For this review, take the finished solid that the model builds, in its own axes (mm). Face numbers are marked on the shaded views. A direction names the side the tool comes from. Round coordinates to 2 decimals unless told otherwise and drop trailing zeros. Write each loop counter-clockwise with the first axis right and the second up, starting at its lowest first coordinate (ties: lowest second). Pieces come first, ordered by that corner, then holes.
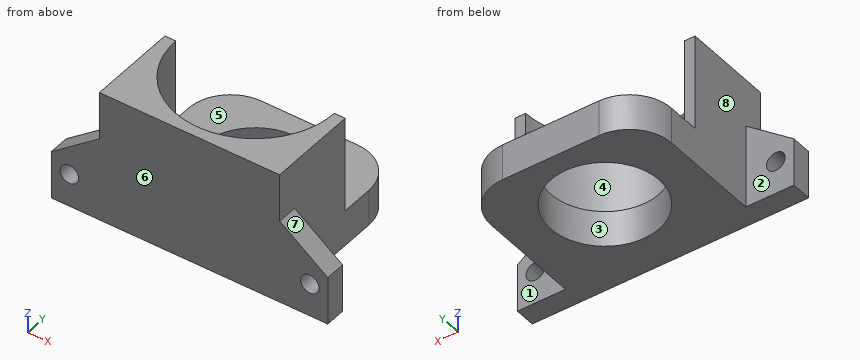
from build123d import *

# Parameters (mm, degrees)
BOSS_EXTRUDE1_DEPTH = 6
SKETCH2_R           = 9
CUT_EXTRUDE1_DEPTH  = 6
FILLET1_R           = 7
BOSS_EXTRUDE2_DEPTH = 16
SKETCH5_W           = 8
SKETCH5_H           = 3.4
BOSS_EXTRUDE3_DEPTH = 2
SKETCH6_R           = 1.55
CUT_EXTRUDE3_DEPTH  = 40.862262856
BOSS_EXTRUDE5_DEPTH = 3.4


with BuildPart() as part:
    # Sketch1 → Boss-Extrude1 (new body)
    with BuildSketch(Plane.XY):
        Polygon((-23, 0), (23, 0), (23, 3.4), (15, 3.4), (15, 27.4), (-15, 27.4), (-15, 3.4), (-23, 3.4), align=None)
    extrude(amount=BOSS_EXTRUDE1_DEPTH)

    # Sketch2 → Cut-Extrude1 (cut)
    with BuildSketch(Plane(origin=(0, 0, 0), x_dir=(-1, 0, 0), z_dir=(0, 0, -1))):
        with Locations((0, 15)):
            Circle(SKETCH2_R)
    extrude(amount=-CUT_EXTRUDE1_DEPTH, mode=Mode.SUBTRACT)

    # Fillet1
    fillet1_edges = [part.edges().sort_by_distance(p)[0] for p in [
        (-15, 27.4, 3),
        (15, 27.4, 3),
    ]]
    fillet(fillet1_edges, radius=FILLET1_R)

    # Sketch4 → Boss-Extrude2 (add)
    with BuildSketch(Plane.XY.offset(6)):
        with BuildLine():
            Line((-15, 0), (15, 0))
            Line((15, 0), (15, 15))
            Line((15, 15), (13.2, 15))
            ThreePointArc((13.2, 15), (0, 1.8), (-13.2, 15))
            Line((-13.2, 15), (-15, 15))
            Line((-15, 15), (-15, 0))
        make_face()
    extrude(amount=BOSS_EXTRUDE2_DEPTH)

    # Sketch5 → Boss-Extrude3 (add)
    with BuildSketch(Plane.XY.offset(6)):
        with Locations((-19, 1.7)):
            Rectangle(SKETCH5_W, SKETCH5_H)
        with Locations((19, 1.7)):
            Rectangle(SKETCH5_W, SKETCH5_H)
    extrude(amount=BOSS_EXTRUDE3_DEPTH)

    # Sketch6 → Cut-Extrude3 (cut, through all)
    with BuildSketch(Plane(origin=(0, 3.4, 0), x_dir=(1, 0, 0), z_dir=(0, 1, 0))):
        with Locations(Location((20, -5.5, 0), (0, 0, 270))):
            Circle(SKETCH6_R)
        with Locations(Location((-20, -5.5, 0), (0, 0, 270))):
            Circle(SKETCH6_R)
    extrude(amount=-CUT_EXTRUDE3_DEPTH, mode=Mode.SUBTRACT)

    # Sketch8 → Boss-Extrude5 (add)
    with BuildSketch(Plane(origin=(0, 0, 0), x_dir=(1, 0, 0), z_dir=(0, 1, 0))):
        Polygon((-23, -8), (-15, -14), (-15, -8), align=None)
        Polygon((15, -14), (23, -8), (15, -8), align=None)
    extrude(amount=BOSS_EXTRUDE5_DEPTH)


solid = part.part
(1) We need section D-D, the plane z = 11. Give the boundary of the cut face in (x, y).
Geometry check:
outline: (-19, 0) - (19, 0) - (19, 3.4) - (15, 3.4) - (15, 15) - (13.2, 15) arc R13.2 cw to (-13.2, 15) - (-15, 15) - (-15, 3.4) - (-19, 3.4) - close
(2) We need section B-B, the plane x = 0. Give the boundary of the cut face in (y, z).
Geometry check:
outline: (0, 0) - (6, 0) - (6, 6) - (1.8, 6) - (1.8, 22) - (0, 22) - close; (24, 0) - (27.4, 0) - (27.4, 6) - (24, 6) - close
(3) For line 1 along X through (y, z) = (2.3, 5.5); line 2 along Y through (x, z) = (-19, 9.5); line 3 along X through (y, z) = (6.75, 4.5), list the stretches that pass through material, from the lowest coordinate up.
Geometry check:
line 1: x = -23 to -21.55, -18.45 to 18.45, 21.55 to 23
line 2: y = 0 to 3.4
line 3: x = -15 to -3.6, 3.6 to 15
(4) Mouldability with a two-part tool opening along X and no side actions: class the marked faces 5, 6, 7 and 8 as pulls with the +X half, pulls with the -X half, needs draft (parallel to the pull), parting line crosses it, or undercut.
Geometry check:
face 5: undercut
face 6: needs draft
face 7: pulls with the +X half
face 8: pulls with the -X half
(5) For the marked faces 1, 2, 3 and 4, list the 3-axis set-ups (+Z, -Z, +X, -X, +Y, -Y) from which the entire face can be reached by the end or side of a thin tool; tool diameter is ignored.
Geometry check:
face 1: +Z, -Z, +X, +Y
face 2: +Z, -Z, -X, +Y
face 3: +Z, -Z
face 4: +Z, +Y
(6) For pin 1 Ø1.4 at (x, z) = (-13.5, 12.5) entering from +Y; pin 2 Ø8 at (x, y) = (-1, 4.5) entering from +Z; pin 3 Ø10 at (y, z) = (13, 12.5) entering from +X; pin 4 Ø11 at (x, y) = (0, 15) entering from -Z, all flat-tipped, find the tip position at first contact; note any pin that passes through.
Geometry check:
pin 1: stops at y = 15
pin 2: stops at z = 22
pin 3: stops at x = 15
pin 4: passes through
(7) We need section C-C, the plane y = 14.5. Give the boundary of the cut face in (x, z).
Geometry check:
outline: (-15, 0) - (-8.99, 0) - (-8.99, 6) - (-13.19, 6) - (-13.19, 22) - (-15, 22) - close; (8.99, 0) - (15, 0) - (15, 22) - (13.19, 22) - (13.19, 6) - (8.99, 6) - close
(8) We need section A-A, the plane z = 5.5. Give the boundary of the cut face in (x, y).
Geometry check:
outline: (-23, 0) - (-21.55, 0) - (-21.55, 3.4) - (-23, 3.4) - close; (-18.45, 0) - (18.45, 0) - (18.45, 3.4) - (15, 3.4) - (15, 20.4) arc R7 ccw to (8, 27.4) - (-8, 27.4) arc R7 ccw to (-15, 20.4) - (-15, 3.4) - (-18.45, 3.4) - close; (21.55, 0) - (23, 0) - (23, 3.4) - (21.55, 3.4) - close; hole circle Ø18 at (0, 15)
